Autodesk Inventor part; units mm, degrees
ref_plane "YZ Plane" through (0, 0, 0) normal (1, 0, 0) x (0, 1, 0)
ref_plane "XZ Plane" through (0, 0, 0) normal (0, 1, 0) x (-1, 0, 0)
ref_plane "XY Plane" through (0, 0, 0) normal (0, 0, 1) x (1, 0, 0)
sketch "Sketch1" plane through (0, 0, 0) normal (0, 1, 0) x (-1, 0, 0)
  point P0 (0, 0)
sketch "Sketch2" plane through (0, 0, 0) normal (0, 1, 0) x (-1, 0, 0)
  circle A0 centre (0, 0) radius 25.5
  dimension "d0" = 51
extrude "Extrusion1" add sketch "Sketch2" along normal blind 2
sketch "Sketch3" plane through (0, 2, 0) normal (0, 1, 0) x (1, 0, 0)
  circle A0 centre (0, 0) radius 22.5
  line L0 (-35.7, 0) -> (35.7, 0)
  line L1 (0, 35.7) -> (0, -35.7)
  point P0 (-22.5, 0)
  point P1 (0, -22.5)
  point P2 (22.5, 0)
  point P3 (0, 22.5)
  dimension "d3" = 45
hole "Hole1" at (-22.5, 2, 0) at (0, 2, 22.5) at (22.5, 2, 0) at (0, 2, -22.5) direction (0, -1, 0) diameter 3 end through all
sketch "Sketch4" plane through (0, 2, 0) normal (0, 1, 0) x (1, 0, 0)
  circle A0 centre (0, 0) radius 10
  point P0 (0, -10)
  point P1 (10, 0)
  point P2 (0, 10)
  point P3 (-10, 0)
  dimension "d11" = 20
hole "Hole2" at (-10, 2, 0) at (0, 2, 10) at (10, 2, 0) at (0, 2, -10) direction (0, -1, 0) diameter 2.459 end through all
properties part number "판"
Verification items for the finished model (mm, model axes). Coordinates: 2 decimals unless noted, no trailing zeros. Order: outer loops, then holes, each group sorted by start corner. A loop starts at its lowest first (then second) coordinate and runs counter-clockwise, first axis right, second up. Notation, with made-up numbers: M 55.25,-32.5 L 61.25,-32.5 A22 cw 61.25,1.5 Z; hole C 56.5,72 d6. An arc over 180 degrees is marked long. Write each question's results on one line, items separated by ' | '.
1) Section check B-B on x = 0. Record the cut outline in (y, z), plus the area to 3 significant figures.
Solved:
outline: M 0,-25.5 L 2,-25.5 L 2,-24 L 0,-24 Z; M 0,-21 L 2,-21 L 2,-11.23 L 0,-11.23 Z; M 0,-8.77 L 2,-8.77 L 2,8.77 L 0,8.77 Z; M 0,11.23 L 2,11.23 L 2,21 L 0,21 Z; M 0,24 L 2,24 L 2,25.5 L 0,25.5 Z | area: 80.2 mm²
2) Release check for a two-part mould opening along X. For faces 1 (the face through (21, 1, 0)), 2 (the face through (0, 0, 0)), 3 (the face through (5.5, 1, 24.9)) record: pulls with the +X half, pulls with the -X half, needs draft (parallel to the pull), parting line crosses it, or undercut.
Solved:
face 1: undercut | face 2: needs draft | face 3: parting line crosses it
3) Section check D-D on y = 0.8. Give the number of separate pieces and of enclosed holes in the cut face, plus the area to 3 significant figures.
Solved:
separate pieces: 1 | enclosed holes: 8 | area: 2,000 mm²
4) Gauge pin test, flat end, axial feed: pin 1 Ø1.5 at (x, z) = (-10, 0) entering from -Y. Record the tip position at first contact, or that the pin passes through.
Solved:
pin 1: passes through
5) Section check A-A on z = -22.5. Record the cut outline in (x, y).
Solved:
outline: M -12,0 L -1.5,0 L -1.5,2 L -12,2 Z; M 1.5,0 L 12,0 L 12,2 L 1.5,2 Z
6) Section check C-C on x = -22.5. Record the cut outline in (y, z).
Solved:
outline: M 0,-12 L 2,-12 L 2,-1.5 L 0,-1.5 Z; M 0,1.5 L 2,1.5 L 2,12 L 0,12 Z
7) Scan lines: line 1 along Z through (x, y) = (0, 1.35); line 2 along X through (y, z) = (1.6, -0.5); line 3 along X through (y, z) = (0.5, -10). Record each from-to range of solid material in increasing order. Write a range as [from, to].
Solved:
line 1: z = [-25.5, -24], [-21, -11.23], [-8.77, 8.77], [11.23, 21], [24, 25.5] | line 2: x = [-25.5, -23.91], [-21.09, -11.12], [-8.88, 8.88], [11.12, 21.09], [23.91, 25.5] | line 3: x = [-23.46, -1.23], [1.23, 23.46]
